Design review of the part built by this model. Coordinates are the model's own, in mm. A direction names the side the tool comes from. Coordinates: 2 decimals unless noted, no trailing zeros. Order: outer loops, then holes, each group sorted by start corner. A loop starts at its lowest first (then second) coordinate and runs counter-clockwise, first axis right, second up. Notation, with made-up numbers: (-28, 84) - (-7, 84) arc R27 ccw to (-7, 115) - close; hole circle Ø7 at (15.5, 72). An arc over 180 degrees is marked (long way). Write item = value, one per line. Start each with the question number.
```python
from build123d import *

# Parameters (mm, degrees)
SKETCH_1_W          = 42.3
SKETCH_1_H          = 42.3
SKETCH_1_R          = 1.75
SKETCH_1_R_2        = 11.25
EXTRUDE_1_DEPTH     = 6
SKETCH_2_W          = 48
SKETCH_2_H          = 42.3
EXTRUDE_2_DEPTH     = 6
SKETCH_3_W          = 48
SKETCH_3_H          = 42.3
EXTRUDE_3_DEPTH     = 6
SKETCH_4_W          = 54.3
SKETCH_4_H          = 48
EXTRUDE_4_DEPTH     = 6
SKETCH_5_W          = 6
SKETCH_5_H          = 6
SKETCH_5_W_2        = 6.359997754
CUT_EXTRUDE_1_DEPTH = 5
SKETCH_6_R          = 2.75
EXTRUDE_5_DEPTH     = 6
SKETCH_7_R          = 2.75
EXTRUDE_6_DEPTH     = 6


with BuildPart() as part:
    # Эскиз1 → Бобышка-Вытянуть1 (new body)
    with BuildSketch(Plane.XY):
        with Locations((21.15, 21.15)):
            Rectangle(SKETCH_1_W, SKETCH_1_H)
        with Locations((36.65, 36.65)):
            Circle(SKETCH_1_R, mode=Mode.SUBTRACT)
        with Locations((5.65, 36.65)):
            Circle(SKETCH_1_R, mode=Mode.SUBTRACT)
        with Locations((5.65, 5.65)):
            Circle(SKETCH_1_R, mode=Mode.SUBTRACT)
        with Locations((36.65, 5.65)):
            Circle(SKETCH_1_R, mode=Mode.SUBTRACT)
        with Locations((21.15, 21.15)):
            Circle(SKETCH_1_R_2, mode=Mode.SUBTRACT)
    extrude(amount=EXTRUDE_1_DEPTH)

    # Эскиз2 → Бобышка-Вытянуть2 (add)
    with BuildSketch(Plane.ZY):
        with Locations((-18, 21.15)):
            Rectangle(SKETCH_2_W, SKETCH_2_H)
    extrude(amount=EXTRUDE_2_DEPTH)

    # Эскиз3 → Бобышка-Вытянуть3 (add)
    with BuildSketch(Plane(origin=(42.3, 0, 0), x_dir=(0, 0, -1), z_dir=(1, 0, 0))):
        with Locations((18, 21.15)):
            Rectangle(SKETCH_3_W, SKETCH_3_H)
    extrude(amount=EXTRUDE_3_DEPTH)

    # Эскиз4 → Бобышка-Вытянуть4 (add)
    with BuildSketch(Plane.XZ):
        with Locations((21.15, -18)):
            Rectangle(SKETCH_4_W, SKETCH_4_H)
    extrude(amount=EXTRUDE_4_DEPTH)

    # Эскиз5 → Вырез-Вытянуть1 (cut)
    with BuildSketch(Plane.XZ.offset(6)):
        with Locations((45.3, -39)):
            Rectangle(SKETCH_5_W, SKETCH_5_H)
        with Locations((-3, -39)):
            Rectangle(SKETCH_5_W, SKETCH_5_H)
        with Locations((-2.820001123, 3)):
            Rectangle(SKETCH_5_W_2, SKETCH_5_H)
        with Locations((45.3, 3)):
            Rectangle(SKETCH_5_W, SKETCH_5_H)
    extrude(amount=-CUT_EXTRUDE_1_DEPTH, mode=Mode.SUBTRACT)

    # Эскиз6 → Бобышка-Вытянуть5 (add)
    with BuildSketch(Plane.XZ.offset(1)):
        with Locations((45.3, 3)):
            Circle(SKETCH_6_R)
    extrude(amount=EXTRUDE_5_DEPTH)

    # Эскиз7 → Бобышка-Вытянуть6 (add)
    with BuildSketch(Plane.XZ.offset(1)):
        with Locations((45.3, -39)):
            Circle(SKETCH_7_R)
    extrude(amount=EXTRUDE_6_DEPTH)


solid = part.part
```
Item 1: Add section C-C on x = 36.65. Give the boundary of the cut face in (y, z), plus the area to 3 significant figures.
Item 2: For faces 4 (the flat face through (45, -4, 0)), 5 (the flat face through (43, -1, 1)), 6 (the flat face through (42.3, -4, 3)), 7 (the flat face through (-3, -4, 0)), list the 3-axis set-ups (+Z, -Z, +X, -X, +Y, -Y) from which the entire face can be reached by the end or side of a thin tool; tool diameter is ignored.
Item 3: Add section B-B on z = 3. Give the boundary of the cut face in (x, y).
Item 4: Mouldability with a two-part tool opening along X and no side actions: class faces 1 (the flat face through (42.3, 21, -21)), 2 (the flat face through (21, 42.3, 2)), 3 (the flat face through (0, -4, -39)) as +X half, -X half, draft (parallel to the pull), parting line (faces both ways), or undercut.
Item 5: Add section D-D on x = 21.15. Give the boundary of the cut face in (y, z).
Item 6: Add section A-A on y = 36.65. Give the boundary of the cut face in (x, z).
Item 7: For P1, Ø1.5, axis at x = 45, y = -3, coming from the -Z side; P2, Ø4, axis at x = 25, z = -18, coming from the -Y side; P3, Ø3, axis at x = -1.5, z = 3.5, coming from the -Y side, all flat-tipped, find the tip position at first contact; note any pin that passes through.
Item 8: For line 1 (Y direction, x = 5.65, z = 3.2); line 2 (X direction, y = 21, z = 3); line 3 (X direction, y = 38, z = -11), list the stretches that pass through material, from the lowest coordinate up.
Worked out:
q1.outline = (-6, -42) - (0, -42) - (0, 0) - (3.9, 0) - (3.9, 6) - (-6, 6) - close; (7.4, 0) - (34.9, 0) - (34.9, 6) - (7.4, 6) - close; (38.4, 0) - (42.3, 0) - (42.3, 6) - (38.4, 6) - close
q1.area = 500 mm2
q2.face_4 = +X, -Y
q2.face_5 = -Y
q2.face_6 = +Z, -Y
q2.face_7 = +Z, -X, -Y
q3.outline = (-6, -1) - (0.36, -1) - (0.36, -6) - (42.3, -6) - (42.3, -1) - (42.55, -1) - (42.55, -7) - (48.05, -7) - (48.05, -1) - (48.3, -1) - (48.3, 42.3) - (-6, 42.3) - close; hole circle Ø3.5 at (5.65, 5.65); hole circle Ø3.5 at (5.65, 36.65); hole circle Ø22.5 at (21.15, 21.15); hole circle Ø3.5 at (36.65, 5.65); hole circle Ø3.5 at (36.65, 36.65)
q4.face_1 = undercut
q4.face_2 = draft
q4.face_3 = -X half
q5.outline = (-6, -42) - (0, -42) - (0, 0) - (9.9, 0) - (9.9, 6) - (-6, 6) - close; (32.4, 0) - (42.3, 0) - (42.3, 6) - (32.4, 6) - close
q6.outline = (-6, -42) - (0, -42) - (0, 0) - (3.9, 0) - (3.9, 6) - (-6, 6) - close; (7.4, 0) - (34.9, 0) - (34.9, 6) - (7.4, 6) - close; (38.4, 0) - (42.3, 0) - (42.3, -42) - (48.3, -42) - (48.3, 6) - (38.4, 6) - close
q7.P1 = -41.75
q7.P2 = -6
q7.P3 = -1
q8.line_1 = -6 to 3.9, 7.4 to 34.9, 38.4 to 42.3
q8.line_2 = -6 to 9.9, 32.4 to 48.3
q8.line_3 = -6 to 0, 42.3 to 48.3
